Read the model definition and answer for the solid it produces. Units are mm, in the model's axes. Face numbers are marked on the shaded views. A direction names the side the tool comes from. Coordinates: 2 decimals unless noted, no trailing zeros. Write each loop counter-clockwise with the first axis right and the second up, starting at its lowest first coordinate (ties: lowest second). Pieces come first, ordered by that corner, then holes.
(1) Section A-A on x = 0 is taken. Write down the section's boundary in (y, z).
(2) Find the intervals of material crossed by probe 1 along Z at (x, y) = (50, 3.1); probe 2 along Y at (x, z) = (16.5, -23); probe 3 along X at (y, z) = (0.85, 0), in increasing order.
(3) Section C-C on y = 14.5 is taken. Write down the section's boundary in (x, z), then the cut area to 3 significant figures.
(4) The mould has two halves that part along Z. Classify the marked faces 1, 2 and 3: +Z half, -Z half, draft (parallel to the pull), parting line (faces both ways), or undercut.
(5) Section B-B on z = 0 is taken. Write down the section's boundary in (x, y).
(6) Given pin 1 (4 mm diameter, centred on x = 50, z = -56, fed in from +Y); pin 2 (5 mm diameter, centred on y = 5.5, z = 22.5, fed in from +X); pin 3 (5 mm diameter, centred on x = 18, z = 8, fed in from +Y); pin 4 (6 mm diameter, centred on y = 26, z = -21, fed in from -X), each flat-ended and moving along its own axis, determine where each tip first touches the part or whether it passes through.
(7) Which of the six approach directions +Z, -Z, +X, -X, +Y, -Y give full straight-line access (tool end or side, diameter ignored) to the marked faces 4, 5, 6 and 7?
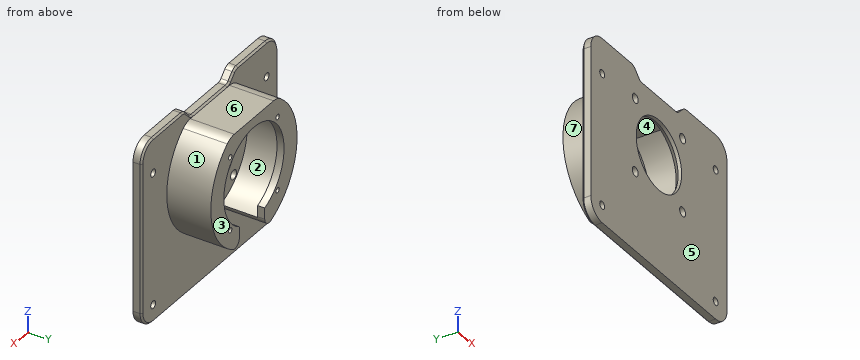
from build123d import *

# Parameters (mm, degrees)
SKETCH2_W           = 120
SKETCH2_H           = 105
BOSS_EXTRUDE2_DEPTH = 5
CUT_EXTRUDE7_DEPTH  = 6
FILLET5_R           = 10
SKETCH10_R          = 20
CUT_EXTRUDE9_DEPTH  = 6
CHAMFER3_SIZE       = 3
FILLET6_R           = 5
CHAMFER4_SIZE       = 1
SKETCH11_R          = 2.15
CUT_EXTRUDE10_DEPTH = 6
BOSS_EXTRUDE3_DEPTH = 25
BOSS_EXTRUDE4_START = -25
SKETCH27_3_R        = 1.45
BOSS_EXTRUDE4_DEPTH = 4
SKETCH28_R          = 2.625
CUT_EXTRUDE13_DEPTH = 5
FILLET7_R           = 10
FILLET8_R           = 4


with BuildPart() as part:
    # Sketch2 → Boss-Extrude2 (new body)
    with BuildSketch(Plane(origin=(0, 0, 0), x_dir=(1, 0, 0), z_dir=(0, 1, 0))):
        with Locations((0, 13.5)):
            Rectangle(SKETCH2_W, SKETCH2_H)
    extrude(amount=BOSS_EXTRUDE2_DEPTH)

    # Sketch9 → Cut-Extrude7 (cut, through all)
    with BuildSketch(Plane(origin=(0, 5, 0), x_dir=(1, 0, 0), z_dir=(0, 1, 0))):
        with BuildLine():
            Line((-17.474873734, -34.025126266), (-23.449747468, -40))
            Line((-23.449747468, -40), (23.449747468, -40))
            Line((23.449747468, -40), (17.474873734, -34.025126266))
            ThreePointArc((17.474873734, -34.025126266), (16.339392013, -33.266421636), (15, -33))
            Line((15, -33), (-15, -33))
            ThreePointArc((-15, -33), (-16.339392013, -33.266421636), (-17.474873734, -34.025126266))
        make_face()
    extrude(amount=-CUT_EXTRUDE7_DEPTH, mode=Mode.SUBTRACT)

    # Fillet5
    fillet5_edges = [part.edges().sort_by_distance(p)[0] for p in [
        (-60, 2.5, -66),
        (60, 2.5, -66),
        (60, 2.5, 39),
        (-60, 2.5, 39),
    ]]
    fillet(fillet5_edges, radius=FILLET5_R)

    # Sketch10 → Cut-Extrude9 (cut, through all)
    with BuildSketch(Plane(origin=(0, 0, 0), x_dir=(1, 0, 0), z_dir=(0, 1, 0))):
        Circle(SKETCH10_R)
    extrude(amount=CUT_EXTRUDE9_DEPTH, mode=Mode.SUBTRACT)

    # Chamfer3
    chamfer3_edges = [part.edges().sort_by_distance(p)[0] for p in [
        (-20, 5, 0),
    ]]
    chamfer(chamfer3_edges, length=CHAMFER3_SIZE)

    # Fillet6
    fillet6_edges = [part.edges().sort_by_distance(p)[0] for p in [
        (22.449747468, 2.5, 39),
        (-22.449747468, 2.5, 39),
    ]]
    fillet(fillet6_edges, radius=FILLET6_R)

    # Chamfer4
    chamfer4_edges = [part.edges().sort_by_distance(p)[0] for p in [
        (16.339392013, 5, 33.266421636),
        (0, 5, 33),
        (-16.339392013, 5, 33.266421636),
        (-19.230077554, 5, 35.780330086),
        (-60, 5, -13.5),
        (0, 5, -66),
        (60, 5, -13.5),
        (-37.26040764, 5, 39),
        (-57.071067812, 5, 36.071067812),
        (57.071067812, 5, 36.071067812),
        (57.071067812, 5, -63.071067812),
        (-57.071067812, 5, -63.071067812),
        (19.230077554, 5, 35.780330086),
        (37.26040764, 5, 39),
        (22.607398118, 5, 38.619397663),
        (-22.607398118, 5, 38.619397663),
    ]]
    chamfer(chamfer4_edges, length=CHAMFER4_SIZE)

    # Sketch11 → Cut-Extrude10 (cut, through all)
    with BuildSketch(Plane(origin=(0, 5, 0), x_dir=(1, 0, 0), z_dir=(0, 1, 0))):
        with Locations((-50, 56)):
            Circle(SKETCH11_R)
        with Locations((50, 56)):
            Circle(SKETCH11_R)
        with Locations((-50, -19)):
            Circle(SKETCH11_R)
        with Locations((50, -19)):
            Circle(SKETCH11_R)
    extrude(amount=-CUT_EXTRUDE10_DEPTH, mode=Mode.SUBTRACT)

    # Sketch27 → Boss-Extrude3 (add)
    with BuildSketch(Plane.XZ.offset(-5)):
        with BuildLine():
            Line((15, 32), (-15, 32))
            Line((-15, 32), (-20.493901532, 32))
            ThreePointArc((-20.493901532, 32), (-37.525010245, -5.989457917), (-9.514215685, -36.789668385))
            Line((-9.514215685, -36.789668385), (-9.514215685, -31.598729403))
            ThreePointArc((-9.514215685, -31.598729403), (-32.683633122, -4.55852234), (-17.797335541, 27.789473684))
            Line((-17.797335541, 27.789473684), (17.797335541, 27.789473684))
            ThreePointArc((17.797335541, 27.789473684), (32.881527048, -2.793775048), (12.853805326, -30.393744235))
            Line((12.853805326, -30.393744235), (12.853805326, -35.760029204))
            ThreePointArc((12.853805326, -35.760029204), (37.760730628, -4.257607592), (20.493901532, 32))
            Line((20.493901532, 32), (15, 32))
        make_face()
    extrude(amount=-BOSS_EXTRUDE3_DEPTH)

    # Sketch27<3> → Boss-Extrude4 (add)
    with BuildSketch(Plane.XZ.offset(-5).offset(BOSS_EXTRUDE4_START)):
        with BuildLine():
            ThreePointArc((-17.797335541, 27.789473684), (-32.683633122, -4.55852234), (-9.514215685, -31.598729403))
            Line((-9.514215685, -31.598729403), (-9.514215685, -24.786250802))
            ThreePointArc((-9.514215685, -24.786250802), (-1.842083043, 26.485566994), (12.853805326, -23.230544926))
            Line((12.853805326, -23.230544926), (12.853805326, -30.393744235))
            ThreePointArc((12.853805326, -30.393744235), (32.881527048, -2.793775048), (17.797335541, 27.789473684))
            Line((17.797335541, 27.789473684), (-17.797335541, 27.789473684))
        make_face()
        with Locations((-20.859650045, -20.859650045)):
            Circle(SKETCH27_3_R, mode=Mode.SUBTRACT)
        with Locations((20.859650045, -20.859650045)):
            Circle(SKETCH27_3_R, mode=Mode.SUBTRACT)
        with Locations((-20.859650045, 20.859650045)):
            Circle(SKETCH27_3_R, mode=Mode.SUBTRACT)
        with Locations((20.859650045, 20.859650045)):
            Circle(SKETCH27_3_R, mode=Mode.SUBTRACT)
    extrude(amount=BOSS_EXTRUDE4_DEPTH)

    # Sketch28 → Cut-Extrude13 (cut)
    with BuildSketch(Plane.XZ):
        with Locations((-20.859650045, 20.859650045)):
            Circle(SKETCH28_R)
        with Locations((20.859650045, 20.859650045)):
            Circle(SKETCH28_R)
        with Locations((20.859650045, -20.859650045)):
            Circle(SKETCH28_R)
        with Locations((-20.859650045, -20.859650045)):
            Circle(SKETCH28_R)
    extrude(amount=-CUT_EXTRUDE13_DEPTH, mode=Mode.SUBTRACT)

    # Fillet7
    fillet7_edges = [part.edges().sort_by_distance(p)[0] for p in [
        (-20.493901532, 17.5, 32),
        (20.493901532, 17.5, 32),
    ]]
    fillet(fillet7_edges, radius=FILLET7_R)

    # Fillet8
    fillet8_edges = [part.edges().sort_by_distance(p)[0] for p in [
        (-9.514215685, 17.5, -36.789668385),
        (12.853805326, 17.5, -35.760029204),
    ]]
    fillet(fillet8_edges, radius=FILLET8_R)


solid = part.part
Response:
1. outline: (0, -66) - (4, -66) - (5, -65) - (5, -23) - (2, -20) - (0, -20) - close; (0, 20) - (2, 20) - (5, 23) - (5, 27.79) - (26, 27.79) - (26, 26.55) - (30, 26.55) - (30, 32) - (5, 32) - (4, 33) - (0, 33) - close
2. probe 1: z = -66 to -58.15, -53.85 to 16.85, 21.15 to 39
2. probe 2: y = 0 to 5, 26 to 30
2. probe 3: x = -60 to -20, 20 to 60
3. outline: (-23.51, 29.86) arc R38 ccw to (-15.1, -34.87) arc R4 ccw to (-9.53, -31.59) arc R33 cw to (-17.8, 27.79) - (17.8, 27.79) arc R33 cw to (12.94, -30.36) arc R4 ccw to (18.84, -33) arc R38 ccw to (23.51, 29.86) arc R10 ccw to (17.32, 32) - (-17.32, 32) arc R10 ccw to start
3. area: 941 mm2
4. face 1: parting line
4. face 2: undercut
4. face 3: draft
5. outline: (-60, 0) - (-20, 0) - (-20, 2) - (-23, 5) - (-33, 5) - (-33, 26) - (-26.55, 26) - (-26.55, 30) - (-38, 30) - (-38, 5) - (-59, 5) - (-60, 4) - close; (20, 0) - (60, 0) - (60, 4) - (59, 5) - (38, 5) - (38, 30) - (26.55, 30) - (26.55, 26) - (33, 26) - (33, 5) - (23, 5) - (20, 2) - close
6. pin 1: passes through
6. pin 2: stops at x = 60
6. pin 3: stops at y = 4.2
6. pin 4: stops at x = -33.47
7. face 4: none
7. face 5: +Z, -Z, +X, -X, -Y
7. face 6: +Z, +X, -X, +Y
7. face 7: -X, +Y
